Source: CAD feature listing. Evaluate the final solid. Frame: model axes, mm. Round coordinates to 2 decimals unless told otherwise and drop trailing zeros. Write each loop counter-clockwise with the first axis right and the second up, starting at its lowest first coordinate (ties: lowest second). Pieces come first, ordered by that corner, then holes. Notation, with made-up numbers: M 19,66.5 L 46,66.5 A23 cw 46,88.5 Z; hole C 3,-33 d7. An arc over 180 degrees is marked long. Answer in a Markdown table with one row per item. Add a question column.
Item 1: Cut plane B-B on x = 3.9. Return loops of the section in (y, z), and give its area (3 significant figures).
Item 2: Contact query for flat-ended pins moving along their axis: pin 1 (5.5 mm diameter, centred on y = 133.242, z = -123.706, fed in from +X); pin 2 (1.5 mm diameter, centred on x = 3.5, z = 110.5, fed in from +Y). Output: stop coordinate, or through.
Item 3: Cut plane D-D on y = 113. Return loops of the section in (x, z), and give its area (3 significant figures).
Item 4: Cut plane C-C on z = 199. Return loops of the section in (x, y), and give its area (3 significant figures).
Item 5: Material intervals for probe 1 along Z at (x, y) = (0.65, 64); probe 2 along Y at (x, z) = (4.55, 129); probe 3 along Y at (x, z) = (0.75, -125.5), sorted ascending.
Item 6: Cut plane A-A on y = 57.5. Return loops of the section in (x, z), and give its area (4 significant figures).
Autodesk Inventor part; units mm, degrees
ref_plane "YZ Plane" through (0, 0, 0) normal (1, 0, 0) x (0, 1, 0)
ref_plane "XZ Plane" through (0, 0, 0) normal (0, 1, 0) x (-1, 0, 0)
ref_plane "XY Plane" through (0, 0, 0) normal (0, 0, 1) x (1, 0, 0)
sketch "スケッチ1" plane through (0, 0, 0) normal (1, 0, 0) x (0, 1, 0)
  line L0 (0, 268.5) -> (0, -268.5)
  line L1 (0, -268.5) -> (175, -268.5)
  line L2 (175, -268.5) -> (175, -48.1515)
  line L3 (175, -48.1515) -> (80, 268.5)
  line L4 (80, 268.5) -> (0, 268.5)
  circle A0 centre (35.142, 228.391) radius 4.1
  circle A1 centre (30.426, 117.793) radius 4.1
  circle A2 centre (83.157, -37.222) radius 3.05
  circle A3 centre (104.738, -109.112) radius 3.05
  circle A4 centre (133.242, -123.706) radius 3.05
  line L5 (65, 128.5) -> (50, 128.5)
  line L6 (50, 128.5) -> (50, 98.5)
  line L7 (50, 98.5) -> (65, 98.5)
  line L8 (65, 98.5) -> (65, 128.5)
  point P0 (0, 0)
  point P1 (0, 0)
  dimension "d0" = 537
  dimension "d1" = 175
  dimension "d2" = 80
  dimension "d3" = 16.7
  dimension "d4" = 40.109
  dimension "d5" = 35.142
  dimension "d6" = 8.2
  dimension "d7" = 150.707
  dimension "d8" = 30.426
  dimension "d9" = 8.2
  dimension "d10" = 305.722
  dimension "d11" = 83.157
  dimension "d12" = 377.612
  dimension "d13" = 104.738
  dimension "d14" = 6.1
  dimension "d15" = 6.1
  dimension "d16" = 133.242
  dimension "d17" = 392.206
  dimension "d18" = 6.1
  dimension "d19" = 140
  dimension "d20" = 50
  dimension "d21" = 30
  dimension "d22" = 15
extrude "押し出し1" add sketch "スケッチ1" along normal blind 5
Results below:
| question | item | result |
|---|---|---|
| 1 | outline | M 0,-268.5 L 175,-268.5 L 175,-48.15 L 80,268.5 L 0,268.5 Z; hole C 30.43,117.79 d8.2; hole C 35.14,228.39 d8.2; hole M 50,98.5 L 65,98.5 L 65,128.5 L 50,128.5 Z; hole C 83.16,-37.22 d6.1; hole C 104.74,-109.11 d6.1; hole C 133.24,-123.71 d6.1 |
| 1 | area | 78,300 mm2 |
| 2 | pin 1 | through |
| 2 | pin 2 | y = 127.63 |
| 3 | outline | M 0,-268.5 L 5,-268.5 L 5,158.51 L 0,158.51 Z |
| 3 | area | 2,140 mm2 |
| 4 | outline | M 0,0 L 5,0 L 5,100.85 L 0,100.85 Z |
| 4 | area | 504 mm2 |
| 5 | probe 1 | -268.5 to 98.5, 128.5 to 268.5 |
| 5 | probe 2 | 0 to 121.85 |
| 5 | probe 3 | 0 to 130.78, 135.71 to 175 |
| 6 | outline | M 0,-268.5 L 5,-268.5 L 5,98.5 L 0,98.5 Z; M 0,128.5 L 5,128.5 L 5,268.5 L 0,268.5 Z |
| 6 | area | 2,535 mm2 |
